Source: CAD feature listing. Evaluate the final solid. Frame: model axes, mm. A direction names the side the tool comes from. Give positions to 0.01 mm unless a question says otherwise; leave off trailing zeros. Write each loop counter-clockwise with the first axis right and the second up, starting at its lowest first coordinate (ties: lowest second). Pieces come first, ordered by that corner, then holes. Notation, with made-up numbers: (48.25, 57) -> (102.25, 57) arc R6 ccw to (102.25, 63) -> close; hole circle Ø10 at (-3.5, 28.5). An arc over 180 degrees is marked (long way). Use one line per item in the form item = value. Start each with the question number.
(1) Cut plane A-A, the plane z = 8. Output: boundary loops of the cut face in (x, y) (3 decimals).
(2) Draft query along Y for faces 4 (the face through (22.383, -4.129, 6.261)), 5 (the face through (-21.695, -5.321, 6.261)), 6 (the face through (0, 9.525, 2)), 7 (the face through (24.13, 0, 19)). Return one class per face: pulls with the +Y half, pulls with the -Y half, needs draft (parallel to the pull), parting line crosses it, or undercut.
(3) Cut plane B-B, the plane z = 25.4. Output: boundary loops of the cut face in (x, y) (3 decimals).
(4) Set-up query: faces 1 (the face through (-24.13, 0, 19)), 2 (the face through (-19, -3, 12.7)), 3 (the face through (-12.7, 0, 22)). Return all of +Z, -Z, +X, -X, +Y, -Y with unobstructed straight access to the full face (end or side cutting, diameter ignored); none if empty.
(5) Material intervals for line 1 along Z through (x, y) = (-15.5, 0) (3 decimals); line 2 along X through (y, z) = (-7, 11.5); line 3 along Z through (x, y) = (-11, 4), sorted ascending. Write a range as from..to.
(6) Cut plane D-D, the plane z = 35.5. Output: boundary loops of the cut face in (x, y) (3 decimals), and give its area (3 significant figures).
(7) First-contact query: P1, Ø8.5, axis at x = 19.35, y = -3.18, coming from the -Z side; P2, Ø3, axis at x = 18.5, y = -3.5, coming from the -Z side; P3, Ø6, axis at x = -7, y = -7, coming from the +Z side. Flat tips, straight axial feed; report the tip coordinate or a pass-through.
(8) Cut plane C-C, the plane y = 1.5. Output: boundary loops of the cut face in (x, z), and give its area (3 significant figures).
from build123d import *

# Parameters (mm, degrees)
F1_DEPTH = 9.525
F2_R     = 3.175
F3_DEPTH = 59.182
F4_R     = 3.175
F5_DEPTH = 12.7


with BuildPart() as f1:
    # F0 (on Front) → F1 (new body, symmetric)
    with BuildSketch(Plane.XZ):
        Polygon((-24.13, 0), (0, 0), (24.13, 0), (24.13, 38.1), (12.7, 38.1), (12.7, 6.35), (0, 6.35), (-12.7, 6.35), (-12.7, 38.1), (-24.13, 38.1), align=None)
    extrude(amount=F1_DEPTH, both=True)

    # F2 (on face) → F3 (cut)
    with BuildSketch(Plane.YZ.offset(24.13)):
        with Locations((0, 25.4)):
            Circle(F2_R)
    extrude(amount=-F3_DEPTH, mode=Mode.SUBTRACT)

    # F4 (on face) → F5 (cut)
    with BuildSketch(Plane(origin=(0, 0, 0), x_dir=(1, 0, 0), z_dir=(0, 0, -1))):
        with Locations((-19.3548, 3.175)):
            Circle(F4_R)
        with Locations((19.3548, 3.175)):
            Circle(F4_R)
    extrude(amount=-F5_DEPTH, mode=Mode.SUBTRACT)


solid = f1.part
Geometry says:
q1.outline = (-24.13, -9.525) -> (-12.7, -9.525) -> (-12.7, 9.525) -> (-24.13, 9.525) -> close; (12.7, -9.525) -> (24.13, -9.525) -> (24.13, 9.525) -> (12.7, 9.525) -> close; hole circle Ø6.35 at (-19.355, -3.175); hole circle Ø6.35 at (19.355, -3.175)
q2.face_4 = undercut
q2.face_5 = undercut
q2.face_6 = pulls with the +Y half
q2.face_7 = needs draft
q3.outline = (-24.13, -9.525) -> (-12.7, -9.525) -> (-12.7, -3.175) -> (-24.13, -3.175) -> close; (-24.13, 3.175) -> (-12.7, 3.175) -> (-12.7, 9.525) -> (-24.13, 9.525) -> close; (12.7, -9.525) -> (24.13, -9.525) -> (24.13, -3.175) -> (12.7, -3.175) -> close; (12.7, 3.175) -> (24.13, 3.175) -> (24.13, 9.525) -> (12.7, 9.525) -> close
q4.face_1 = +Z, -Z, -X, +Y, -Y
q4.face_2 = -Z
q4.face_3 = +Z, +Y, -Y
q5.line_1 = 0..22.225, 28.575..38.1
q5.line_2 = -24.13..-12.7, 12.7..24.13
q5.line_3 = 0..6.35
q6.outline = (-24.13, -9.525) -> (-12.7, -9.525) -> (-12.7, 9.525) -> (-24.13, 9.525) -> close; (12.7, -9.525) -> (24.13, -9.525) -> (24.13, 9.525) -> (12.7, 9.525) -> close
q6.area = 435 mm^2
q7.P1 = 0
q7.P2 = 12.7
q7.P3 = 6.35
q8.outline = (-24.13, 0) -> (24.13, 0) -> (24.13, 22.6) -> (12.7, 22.6) -> (12.7, 6.35) -> (-12.7, 6.35) -> (-12.7, 22.6) -> (-24.13, 22.6) -> close; (-24.13, 28.2) -> (-12.7, 28.2) -> (-12.7, 38.1) -> (-24.13, 38.1) -> close; (12.7, 28.2) -> (24.13, 28.2) -> (24.13, 38.1) -> (12.7, 38.1) -> close
q8.area = 904 mm^2
